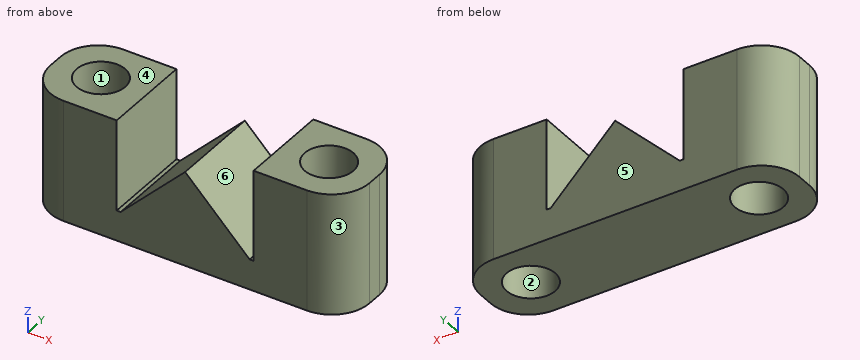
from build123d import *

# Parameters (mm, degrees)
SKETCH1_R           = 1.6
BOSS_EXTRUDE1_DEPTH = 8
SKETCH2_W           = 9
SKETCH2_H           = 8.199711987
CUT_EXTRUDE1_DEPTH  = 8
BOSS_EXTRUDE2_DEPTH = 6


with BuildPart() as part:
    # Sketch1 → Boss-Extrude1 (new body)
    with BuildSketch(Plane.XY):
        with BuildLine():
            Line((-0.5, 3), (15.5, 3))
            ThreePointArc((15.5, 3), (17.267766953, 2.267766953), (18, 0.5))
            Line((18, 0.5), (18, -0.5))
            ThreePointArc((18, -0.5), (17.267766953, -2.267766953), (15.5, -3))
            Line((15.5, -3), (-0.5, -3))
            ThreePointArc((-0.5, -3), (-2.267766953, -2.267766953), (-3, -0.5))
            Line((-3, -0.5), (-3, 0.5))
            ThreePointArc((-3, 0.5), (-2.267766953, 2.267766953), (-0.5, 3))
        make_face()
        Circle(SKETCH1_R, mode=Mode.SUBTRACT)
        with Locations((15, 0)):
            Circle(SKETCH1_R, mode=Mode.SUBTRACT)
    extrude(amount=BOSS_EXTRUDE1_DEPTH)

    # Sketch2 → Cut-Extrude1 (cut)
    with BuildSketch(Plane.XZ.offset(3)):
        with Locations((7.5, 6.099855994)):
            Rectangle(SKETCH2_W, SKETCH2_H)
    extrude(amount=-CUT_EXTRUDE1_DEPTH, mode=Mode.SUBTRACT)

    # Sketch3 → Boss-Extrude2 (add)
    with BuildSketch(Plane.XZ.offset(3)):
        Polygon((3.257359313, 2), (7.5, 6.242640687), (11.742640687, 2), align=None)
    extrude(amount=-BOSS_EXTRUDE2_DEPTH)


solid = part.part
Can you work these out from the model? Positions are in its coordinate system, mm. Face numbers are marked on the shaded views. A direction names the side the tool comes from. Give positions to 0.01 mm unless a question says otherwise; leave off trailing zeros. Loops run counter-clockwise (first coordinate to the right, second up) from the corner with the lowest first, then second, coordinate; pieces in that order, holes last. Notation, with made-up numbers: (5, 80.25) -> (29, 80.25) arc R6 cw to (29, 86.25) -> close; hole circle Ø11 at (-7, -11.5). An arc over 180 degrees is marked (long way). Return JSON: item names as keys, results as strings.
Q1. I want a section at C-C, the plane z = 3.75. List the corners of the cut face in (x, y) for me.
Checks:
{"outline": "(-3, -0.5) arc R2.5 ccw to (-0.5, -3) -> (3, -3) -> (3, 3) -> (-0.5, 3) arc R2.5 ccw to (-3, 0.5) -> close; (5.01, -3) -> (9.99, -3) -> (9.99, 3) -> (5.01, 3) -> close; (12, -3) -> (15.5, -3) arc R2.5 ccw to (18, -0.5) -> (18, 0.5) arc R2.5 ccw to (15.5, 3) -> (12, 3) -> close; hole circle Ø3.2 at (0, 0); hole circle Ø3.2 at (15, 0)"}
Q2. On a 3-axis mill with a long thin cutter (end or side, diameter ignored), from which of +Z, -Z, +X, -X, +Y, -Y can I reach the whole of each face in a straight line? I mean the marked faces 5 and 6. Say none if no direction works.
Checks:
{"face 5": "+Z, -Z, +X, -X, +Y", "face 6": "+Z, +Y, -Y"}
Q3. We'd pull the mould along Y, two halves only. Please class the marked faces 1, 2, 3 and 4: released by +Y, released by -Y, zero draft, split by the parting line, or undercut.
Checks:
{"face 1": "undercut", "face 2": "undercut", "face 3": "released by -Y", "face 4": "zero draft"}
Q4. For pin 1 Ø2.5 at (x, y) = (15, 0) entering from -Z; pin 2 Ø3 at (x, z) = (5.5, 5.5) entering from -Y, each with a flat end and sliding along its axis, tell me the tip position at first contact or that it passes through.
Checks:
{"pin 1": "passes through", "pin 2": "stops at y = -3"}
Q5. I want a section at B-B, the plane x = 15. List the corners of the cut face in (y, z) for me.
Checks:
{"outline": "(-3, 0) -> (-1.6, 0) -> (-1.6, 8) -> (-3, 8) -> close; (1.6, 0) -> (3, 0) -> (3, 8) -> (1.6, 8) -> close"}
Q6. I need wall thicknesses on probe 1 along X at (y, z) = (0.15, 1.5); probe 2 along X at (y, z) = (-1.8, 6); probe 3 along Y at (x, z) = (0, 4). Which ranges of each line are inside material? Lowest first, please.
Checks:
{"probe 1": "x = -3 to -1.59, 1.59 to 13.41, 16.59 to 18", "probe 2": "x = -2.64 to 3, 7.26 to 7.74, 12 to 17.64", "probe 3": "y = -3 to -1.6, 1.6 to 3"}
Q7. I want a section at D-D, the plane y = 0. List the corners of the cut face in (x, z) for me, then the cut area to 3 significant figures.
Checks:
{"outline": "(-3, 0) -> (-1.6, 0) -> (-1.6, 8) -> (-3, 8) -> close; (1.6, 0) -> (13.4, 0) -> (13.4, 8) -> (12, 8) -> (12, 2) -> (11.74, 2) -> (7.5, 6.24) -> (3.26, 2) -> (3, 2) -> (3, 8) -> (1.6, 8) -> close; (16.6, 0) -> (18, 0) -> (18, 8) -> (16.6, 8) -> close", "area": "80.8 mm2"}
Q8. I want a section at A-A, the plane z = 7.25. List the corners of the cut face in (x, y) for me, then the cut area to 4 significant figures.
Checks:
{"outline": "(-3, -0.5) arc R2.5 ccw to (-0.5, -3) -> (3, -3) -> (3, 3) -> (-0.5, 3) arc R2.5 ccw to (-3, 0.5) -> close; (12, -3) -> (15.5, -3) arc R2.5 ccw to (18, -0.5) -> (18, 0.5) arc R2.5 ccw to (15.5, 3) -> (12, 3) -> close; hole circle Ø3.2 at (0, 0); hole circle Ø3.2 at (15, 0)", "area": "50.55 mm2"}
